```python
from build123d import *

# Parameters (mm, degrees)
SKETCH1_R           = 2.667
BOSS_EXTRUDE1_DEPTH = 10.16
SKETCH7_R           = 4.6355
CUT_EXTRUDE1_DEPTH  = 4.064
SKETCH3_R           = 1.397
CUT_EXTRUDE2_DEPTH  = 1.016
SKETCH8_R           = 1.397
CUT_EXTRUDE3_DEPTH  = 1.016
CUT_EXTRUDE4_START  = -1.016
SKETCH9_R           = 1.397
CUT_EXTRUDE4_DEPTH  = 1.016
FILLET1_R           = 1.27


with BuildPart() as part:
    # Sketch1 → Boss-Extrude1 (new body)
    with BuildSketch(Plane.XY):
        Polygon((0, 57.15), (10.16, 57.15), (10.16, 67.31), (22.86, 67.31), (22.86, 57.15), (33.02, 57.15), (33.02, 0), (0, 0), align=None)
        with Locations((26.67, 15.24)):
            Circle(SKETCH1_R, mode=Mode.SUBTRACT)
    extrude(amount=BOSS_EXTRUDE1_DEPTH)

    # Sketch7 → Cut-Extrude1 (cut)
    with BuildSketch(Plane.XY.offset(10.16)):
        with Locations((26.67, 15.24)):
            Circle(SKETCH7_R)
    extrude(amount=-CUT_EXTRUDE1_DEPTH, mode=Mode.SUBTRACT)

    # Sketch3 → Cut-Extrude2 (cut)
    with BuildSketch(Plane(origin=(0, 0, 10.16), x_dir=(-1, 0, 0), z_dir=(0, 0, -1))):
        with Locations((-16.51, 62.23)):
            Circle(SKETCH3_R)
    extrude(amount=CUT_EXTRUDE2_DEPTH, mode=Mode.SUBTRACT)

    # Sketch8 → Cut-Extrude3 (cut)
    with BuildSketch(Plane(origin=(22.86, 0, 0), x_dir=(0, 0, -1), z_dir=(1, 0, 0))):
        with Locations((-5.08, 62.23)):
            Circle(SKETCH8_R)
    extrude(amount=-CUT_EXTRUDE3_DEPTH, mode=Mode.SUBTRACT)

    # Sketch9 → Cut-Extrude4 (cut)
    with BuildSketch(Plane.ZY.offset(-10.16).offset(CUT_EXTRUDE4_START)):
        with Locations(Location((5.08, 62.23, 0), (0, 0, 180))):
            Circle(SKETCH9_R)
    extrude(amount=CUT_EXTRUDE4_DEPTH, mode=Mode.SUBTRACT)

    # Fillet1
    fillet1_edges = [part.edges().sort_by_distance(p)[0] for p in [
        (33.02, 28.575, 10.16),
        (0, 57.15, 5.08),
        (33.02, 57.15, 5.08),
        (33.02, 0, 5.08),
        (0, 0, 5.08),
        (0, 28.575, 10.16),
        (16.51, 0, 10.16),
    ]]
    fillet(fillet1_edges, radius=FILLET1_R)


solid = part.part
```
Geometry: final body of the model. Coordinates: model frame, mm. A direction names the side the tool comes from. Coordinates: 2 decimals unless noted, no trailing zeros. Loops run counter-clockwise (first coordinate to the right, second up) from the corner with the lowest first, then second, coordinate; pieces in that order, holes last. Notation, with made-up numbers: M -25,-26 L 6,-26 A24 cw 6,5 Z; hole C 64.5,68.25 d8. An arc over 180 degrees is marked long. Put each result on its own line as item: value.
(1) Material intervals for probe 1 along Z at (x, y) = (10.45, 62.23); probe 2 along Y at (x, z) = (26.67, 4.25); probe 3 along X at (y, z) = (63, 4), sorted ascending.
Answer sheet:
probe 1: z = 0 to 3.68, 6.48 to 10.16
probe 2: y = 0 to 12.57, 17.91 to 57.15
probe 3: x = 11.18 to 21.84
(2) First-contact query: pin 1 (1.4 mm diameter, centred on x = 17, y = 62.5, fed in from +Z); pin 2 (4.5 mm diameter, centred on x = 5, z = 4.5, fed in from +Y); pin 3 (3 mm diameter, centred on y = 64.5, z = 3, fed in from +X). Flat tips, straight axial feed; report the tip coordinate or a pass-through.
Answer sheet:
pin 1: stops at z = 9.14
pin 2: stops at y = 57.15
pin 3: stops at x = 22.86
(3) Cut plane C-C on y = 62.23. Return the cut outline in (x, z), then the cut area to 3 significant figures.
Answer sheet:
outline: M 10.16,0 L 22.86,0 L 22.86,3.68 L 21.84,3.68 L 21.84,6.48 L 22.86,6.48 L 22.86,10.16 L 17.91,10.16 L 17.91,9.14 L 15.11,9.14 L 15.11,10.16 L 10.16,10.16 L 10.16,6.48 L 11.18,6.48 L 11.18,3.68 L 10.16,3.68 Z
area: 121 mm^2
(4) Cut plane A-A on x = 26.67. Return the cut outline in (y, z), then the cut area to 3 significant figures.
Answer sheet:
outline: M 0,0 L 12.57,0 L 12.57,6.1 L 10.6,6.1 L 10.6,10.16 L 1.27,10.16 A1.27 ccw 0,8.89 Z; M 17.91,0 L 57.15,0 L 57.15,10.16 L 19.88,10.16 L 19.88,6.1 L 17.91,6.1 Z
area: 510 mm^2
(5) Cut plane D-D on x = 9. Return the cut outline in (y, z).
Answer sheet:
outline: M 0,0 L 57.15,0 L 57.15,10.16 L 1.27,10.16 A1.27 ccw 0,8.89 Z
(6) Access query for faces 4 (the face through (22.04, 15.44, 8.16)), 5 (the face through (22.359, 60.866, 5.383)), 6 (the face through (6, 57.15, 5)), 7 (the face through (11.176, 62, 5)). Directions: +Z, -Z, +X, -X, +Y, -Y. A direction counts if a zero-diameter tool reaches every point of the face in a straight line with its end or side. Return the directions, or none.
Answer sheet:
face 4: +Z
face 5: +X
face 6: +Z, -Z, -X, +Y
face 7: -X
(7) Cut plane B-B on z = 5.08. Return the cut outline in (x, y), then the cut area to 3 significant figures.
Answer sheet:
outline: M 0,1.27 A1.27 ccw 1.27,0 L 31.75,0 A1.27 ccw 33.02,1.27 L 33.02,55.88 A1.27 ccw 31.75,57.15 L 22.86,57.15 L 22.86,60.83 L 21.84,60.83 L 21.84,63.63 L 22.86,63.63 L 22.86,67.31 L 10.16,67.31 L 10.16,63.63 L 11.18,63.63 L 11.18,60.83 L 10.16,60.83 L 10.16,57.15 L 1.27,57.15 A1.27 ccw 0,55.88 Z; hole C 26.67,15.24 d5.33
area: 1,990 mm^2
(8) Draft query along Y for faces 1 (the face through (32.638, 0.362, 4.507)), 2 (the face through (10.16, 61, 4)), 3 (the face through (29.134, 14.219, 3.005)). Return one class per face: pulls with the +Y half, pulls with the -Y half, needs draft (parallel to the pull), parting line crosses it, or undercut.
Answer sheet:
face 1: pulls with the -Y half
face 2: needs draft
face 3: undercut
